Part model, mm, in its own coordinate system. A direction names the side the tool comes from. Round coordinates to 2 decimals unless told otherwise and drop trailing zeros. Write each loop counter-clockwise with the first axis right and the second up, starting at its lowest first coordinate (ties: lowest second). Pieces come first, ordered by that corner, then holes.
from build123d import *

# Parameters (mm, degrees)
SKETCH1_W                        = 15
SKETCH1_H                        = 6
MAIN_BODY_EXT_DEPTH              = 8.3
EMISSION_PATH_EXT_DEPTH          = 9
SKETCH3_R                        = 1.25
EMISSION_AND_GRIN_CUT_DEPTH      = 20.092931
SKETCH4_R                        = 1
DRUM_LENS_CUT_DEPTH              = 13
SKETCH41_R                       = 1
ADDTL_LIGHT_SOURCE_DEPTH         = 5
SKETCH5_W                        = 15
SKETCH5_H                        = 7.3
FILTERCOVER_CUT1_DEPTH           = 1
TOP_LED_SCREW_W                  = 3.06
TOP_LED_SCREW_H                  = 2
BOSS_EXTRUDE1_DEPTH              = 1
FILTERSET_CUT2_DEPTH             = 4
SKETCH10_R                       = 2.5
EMISSION_LENS_CUT_DEPTH          = 8.5
SKETCH15_R                       = 0.795
MAGNETS_CUT_DEPTH                = 0.9
SCREW_HOLES_CUT_DEPTH            = 20.507434
SCREW_HOLES_CUT_DEPTH_BACK       = 2.5
SKETCH18_R                       = 0.375
EXTERNAL_FILLET_1_R              = 1.5
VERTICAL_PATH_CUT_DEPTH          = 14.011149
VERTICAL_PATH_CUT_DEPTH_BACK     = 4
SKETCH28_R                       = 1.5
SET_SCREW_NOTCH_DEPTH            = 3
CUT_EXTRUDE_ORIGINAL_LIGHT_DEPTH = 0.7
CUT_EXTRUDE_ADDTL_LIGHT_DEPTH    = 0.7
SKETCH29_R                       = 0.375
SIDE_LED_SCREW_DEPTH             = 2.5
SKETCH32_W                       = 2
SKETCH32_H                       = 2.36
SIDE_WIRE_SLOT_CUT_DEPTH         = 0.7
SKETCH45_W                       = 2.36
SKETCH45_H                       = 2
TOP_LED_SLOT_DEPTH               = 0.7
CUT_EXTRUDE16_DEPTH              = 9
CUT_EXTRUDE17_REACH              = 13.945
SKETCH37_R                       = 2
SKETCH48_R                       = 0.5
PEG_EXTRUDE_DEPTH                = 2
SKETCH51_R                       = 0.375
TOP_LE_SCREW_DEPTH               = 2.1


with BuildPart() as part:
    # Sketch1 → Main Body Ext (new body)
    with BuildSketch(Plane(origin=(0, 0, 0), x_dir=(1, 0, 0), z_dir=(0, 1, 0))):
        Rectangle(SKETCH1_W, SKETCH1_H)
    extrude(amount=MAIN_BODY_EXT_DEPTH)

    # Sketch8 → Emission Path Ext (add)
    with BuildSketch(Plane(origin=(0, 8.3, 0), x_dir=(1, 0, 0), z_dir=(0, 1, 0))):
        Polygon((-2.75, 3), (-1.5, 1.75), (-1.5, -3), (-7.5, -3), (-7.5, 3), align=None)
    extrude(amount=EMISSION_PATH_EXT_DEPTH)

    # Sketch3 → Emission and Grin Cut (cut, through all)
    with BuildSketch(Plane.XZ):
        with Locations(Location((-4.5, 0, 0), (0, 0, 270))):
            Circle(SKETCH3_R)
    extrude(amount=-EMISSION_AND_GRIN_CUT_DEPTH, mode=Mode.SUBTRACT)

    # Sketch4 → Drum Lens Cut (cut)
    with BuildSketch(Plane(origin=(7.5, 0, 0), x_dir=(0, 0, -1), z_dir=(1, 0, 0))):
        with Locations((0, 3)):
            Circle(SKETCH4_R)
    extrude(amount=-DRUM_LENS_CUT_DEPTH, mode=Mode.SUBTRACT)

    # Sketch41 → Addtl Light Source (cut)
    with BuildSketch(Plane(origin=(0, 8.3, 0), x_dir=(1, 0, 0), z_dir=(0, 1, 0))):
        with Locations(Location((1.5, 0, 0), (0, 0, 270))):
            Circle(SKETCH41_R)
    extrude(amount=-ADDTL_LIGHT_SOURCE_DEPTH, mode=Mode.SUBTRACT)

    # Sketch5 → FilterCover Cut1 (cut)
    with BuildSketch(Plane.XY.offset(3)):
        with Locations((0, 4.65)):
            Rectangle(SKETCH5_W, SKETCH5_H)
    extrude(amount=-FILTERCOVER_CUT1_DEPTH, mode=Mode.SUBTRACT)

    # Top-LED-Screw → Boss-Extrude1 (add)
    with BuildSketch(Plane.XY.offset(2)):
        with Locations((5.97, 7.3)):
            Rectangle(TOP_LED_SCREW_W, TOP_LED_SCREW_H)
    extrude(amount=BOSS_EXTRUDE1_DEPTH)

    # Sketch6 → FilterSet Cut2 (cut)
    with BuildSketch(Plane.XY.offset(2)):
        with BuildLine():
            Line((5.3, 4.5), (5.3, 1.8))
            ThreePointArc((5.3, 1.8), (5.7, 1.4), (5.3, 1))
            Line((5.3, 1), (4.1, 1))
            ThreePointArc((4.1, 1), (3.7, 1.4), (4.1, 1.8))
            Line((4.1, 1.8), (4.1, 4.5))
            ThreePointArc((4.1, 4.5), (4.7, 5.1), (5.3, 4.5))
        make_face()
        with BuildLine():
            Line((-6.9, 7.9), (-6.9, 7.5))
            ThreePointArc((-6.9, 7.5), (-6.782843, 7.217157), (-6.5, 7.1))
            Line((-6.5, 7.1), (-2.5, 7.1))
            ThreePointArc((-2.5, 7.1), (-2.217157, 7.217157), (-2.1, 7.5))
            Line((-2.1, 7.5), (-2.1, 7.9))
            ThreePointArc((-2.1, 7.9), (-2.217157, 8.182843), (-2.5, 8.3))
            Line((-2.5, 8.3), (-6.5, 8.3))
            ThreePointArc((-6.5, 8.3), (-6.782843, 8.182843), (-6.9, 7.9))
        make_face()
        with BuildLine():
            Line((-2.605887, 6.591169), (-6.848528, 2.348528))
            ThreePointArc((-6.848528, 2.348528), (-6.848528, 1.5), (-6, 1.5))
            Line((-6, 1.5), (-1.757359, 5.742641))
            ThreePointArc((-1.757359, 5.742641), (-1.757359, 6.591169), (-2.605887, 6.591169))
        make_face()
        with BuildLine():
            Line((3.112092, 6.591169), (-1.130548, 2.348528))
            ThreePointArc((-1.130548, 2.348528), (-1.130548, 1.5), (-0.28202, 1.5))
            Line((-0.28202, 1.5), (3.96062, 5.742641))
            ThreePointArc((3.96062, 5.742641), (3.96062, 6.591169), (3.112092, 6.591169))
        make_face()
    extrude(amount=-FILTERSET_CUT2_DEPTH, mode=Mode.SUBTRACT)

    # Sketch10 → Emission Lens Cut (cut)
    with BuildSketch(Plane(origin=(0, 17.3, 0), x_dir=(1, 0, 0), z_dir=(0, 1, 0))):
        with Locations(Location((-4.5, 0, 0), (0, 0, 270))):
            Circle(SKETCH10_R)
    extrude(amount=-EMISSION_LENS_CUT_DEPTH, mode=Mode.SUBTRACT)

    # Sketch15 → Magnets Cut (cut)
    with BuildSketch(Plane.XZ):
        with Locations(Location((-6.25, -1.875, 0), (0, 0, 270))):
            Circle(SKETCH15_R)
        with Locations(Location((-6.25, 1.875, 0), (0, 0, 270))):
            Circle(SKETCH15_R)
        with Locations(Location((-1.5, 0, 0), (0, 0, 270))):
            Circle(SKETCH15_R)
    extrude(amount=-MAGNETS_CUT_DEPTH, mode=Mode.SUBTRACT)

    # Sketch18 → Screw Holes Cut (cut, two sides: drawn at the far end of the back side and taken through both)
    with BuildSketch(Plane.XY.offset(2).offset(-SCREW_HOLES_CUT_DEPTH_BACK)):
        with Locations(Location((-6.5, 4, 0), (0, 0, 180))):
            Circle(SKETCH18_R)
        with Locations(Location((6, 5.8, 0), (0, 0, 180))):
            Circle(SKETCH18_R)
        with Locations((0.25, 1)):
            Circle(SKETCH18_R)
    extrude(amount=SCREW_HOLES_CUT_DEPTH + SCREW_HOLES_CUT_DEPTH_BACK, mode=Mode.SUBTRACT)

    # External Fillet 1
    # the kernel refuses this fillet: 1.5 mm, written as the material it takes off along each edge
    with BuildSketch(Plane(origin=(-7.5, -3.75, -3), x_dir=(1, 0, 0), z_dir=(0, 1, 0))) as external_fillet_1_piece_1:
        with BuildLine():
            CenterArc((EXTERNAL_FILLET_1_R, -EXTERNAL_FILLET_1_R), EXTERNAL_FILLET_1_R, 90, 90)
            Line((0, -EXTERNAL_FILLET_1_R), (0, 0))
            Line((0, 0), (EXTERNAL_FILLET_1_R, 0))
        make_face()
    extrude(amount=24.8, mode=Mode.SUBTRACT)
    with BuildSketch(Plane(origin=(-1.5, 8.3, 3), x_dir=(0, 0, -1), z_dir=(0, 1, 0))) as external_fillet_1_piece_2:
        with BuildLine():
            CenterArc((EXTERNAL_FILLET_1_R, EXTERNAL_FILLET_1_R), EXTERNAL_FILLET_1_R, 180, 90)
            Line((0, EXTERNAL_FILLET_1_R), (0, 0))
            Line((0, 0), (EXTERNAL_FILLET_1_R, 0))
        make_face()
    extrude(amount=12.75, mode=Mode.SUBTRACT)

    # Sketch28 → Vertical-Path-Cut (cut, two sides: drawn at the far end of the back side and taken through both)
    with BuildSketch(Plane(origin=(0, 7.1, 0), x_dir=(1, 0, 0), z_dir=(0, 1, 0)).offset(-VERTICAL_PATH_CUT_DEPTH_BACK)):
        with Locations(Location((-4.5, 0, 0), (0, 0, 180))):
            Circle(SKETCH28_R)
    extrude(amount=VERTICAL_PATH_CUT_DEPTH + VERTICAL_PATH_CUT_DEPTH_BACK, mode=Mode.SUBTRACT)

    # Sketch14 → Set-Screw-Notch (cut)
    with BuildSketch(Plane.XZ):
        Polygon((7.5, -3), (7.5, -1.891585), (7.056634, -3), align=None)
    extrude(amount=-SET_SCREW_NOTCH_DEPTH, mode=Mode.SUBTRACT)

    # Sketch12 → Cut-Extrude Original Light (cut)
    with BuildSketch(Plane(origin=(7.5, 0, 0), x_dir=(0, 0, -1), z_dir=(1, 0, 0))):
        with BuildLine():
            Line((1.6, 5.94), (-1.6, 5.94))
            Line((-1.6, 5.94), (-2, 5.94))
            Line((-2, 5.94), (-2, 1.33))
            Line((-2, 1.33), (1.6, 1.33))
            ThreePointArc((1.6, 1.33), (1.882843, 1.447157), (2, 1.73))
            Line((2, 1.73), (2, 5.54))
            ThreePointArc((2, 5.54), (1.882843, 5.822843), (1.6, 5.94))
        make_face()
    extrude(amount=-CUT_EXTRUDE_ORIGINAL_LIGHT_DEPTH, mode=Mode.SUBTRACT)

    # Sketch44 → Cut-Extrude Addtl Light (cut)
    with BuildSketch(Plane(origin=(0, 8.3, 0), x_dir=(1, 0, 0), z_dir=(0, 1, 0))):
        with BuildLine():
            Line((-0.17, -2), (4.44, -2))
            Line((4.44, -2), (4.44, 1.6))
            ThreePointArc((4.44, 1.6), (4.322843, 1.882843), (4.04, 2))
            Line((4.04, 2), (0.23, 2))
            ThreePointArc((0.23, 2), (-0.052843, 1.882843), (-0.17, 1.6))
            Line((-0.17, 1.6), (-0.17, -2))
        make_face()
    extrude(amount=-CUT_EXTRUDE_ADDTL_LIGHT_DEPTH, mode=Mode.SUBTRACT)

    # Sketch29 → Side-LED-Screw (cut)
    with BuildSketch(Plane(origin=(7.5, 0, 0), x_dir=(0, 0, -1), z_dir=(1, 0, 0))):
        with Locations((2, 6.5)):
            Circle(SKETCH29_R)
    extrude(amount=-SIDE_LED_SCREW_DEPTH, mode=Mode.SUBTRACT)

    # Sketch32 → Side-Wire-Slot-Cut (cut)
    with BuildSketch(Plane(origin=(7.5, 0, 0), x_dir=(0, 0, -1), z_dir=(1, 0, 0))):
        with Locations((0, 7.12)):
            Rectangle(SKETCH32_W, SKETCH32_H)
    extrude(amount=-SIDE_WIRE_SLOT_CUT_DEPTH, mode=Mode.SUBTRACT)

    # Sketch45 → Top-LED-slot (cut)
    with BuildSketch(Plane(origin=(0, 8.3, 0), x_dir=(1, 0, 0), z_dir=(0, 1, 0))):
        with Locations((5.62, 0)):
            Rectangle(SKETCH45_W, SKETCH45_H)
    extrude(amount=-TOP_LED_SLOT_DEPTH, mode=Mode.SUBTRACT)

    # Sketch33 → Side-BallLens_Cut (revolve, cut)
    with BuildSketch(Plane.XY, mode=Mode.PRIVATE) as side_balllens_cut_sk:
        with BuildLine():
            Line((6.8, 3), (5.3, 3))
            ThreePointArc((5.3, 3), (5.73934, 4.06066), (6.8, 4.5))
            Line((6.8, 4.5), (6.8, 3))
        make_face()
    revolve(side_balllens_cut_sk.sketch.rotate(Axis((6.8, 3, 0), (-1, 0, 0)), 84.26086), axis=Axis((6.8, 3, 0), (-1, 0, 0)), mode=Mode.SUBTRACT)

    # Sketch47 → Top-BallLens_Cut (revolve, cut)
    with BuildSketch(Plane(origin=(1.5, 0, 0), x_dir=(0, 0, -1), z_dir=(1, 0, 0))):
        with BuildLine():
            Line((-1.5, 7.6), (0, 7.6))
            Line((0, 7.6), (0, 6.137287))
            ThreePointArc((0, 6.137287), (-1.04756, 6.563498), (-1.5, 7.6))
        make_face()
    revolve(axis=Axis((1.5, 7.6, 0), (0, -1, 0)), mode=Mode.SUBTRACT)

    # Sketch36 → Cut-Extrude16 (cut)
    with BuildSketch(Plane(origin=(0, 17.3, 0), x_dir=(1, 0, 0), z_dir=(0, 1, 0))):
        with BuildLine():
            Line((-7.5, -1.5), (-7.5, -3))
            Line((-7.5, -3), (-6, -3))
            ThreePointArc((-6, -3), (-7.06066, -2.56066), (-7.5, -1.5))
        make_face()
    extrude(amount=-CUT_EXTRUDE16_DEPTH, mode=Mode.SUBTRACT)

    # Sketch37 → Cut-Extrude17 (cut, up to next)
    with BuildSketch(Plane(origin=(0, 8.8, 0), x_dir=(1, 0, 0), z_dir=(0, 1, 0)), mode=Mode.PRIVATE) as cut_extrude17_sk1:
        with Locations(Location((-4.5, 0, 0), (0, 0, 180))):
            Circle(SKETCH37_R)
    cut_extrude17_tool1 = extrude(cut_extrude17_sk1.sketch, amount=-CUT_EXTRUDE17_REACH, mode=Mode.PRIVATE) & part.part
    add(cut_extrude17_tool1.solids().sort_by_distance((-4.5, 8.8, 0))[0], mode=Mode.SUBTRACT)

    # Sketch48 → Peg-extrude (cut)
    with BuildSketch(Plane.XZ):
        with Locations(Location((-2, -2, 0), (0, 0, 270))):
            Circle(SKETCH48_R)
    extrude(amount=-PEG_EXTRUDE_DEPTH, mode=Mode.SUBTRACT)

    # Sketch51 → Top-LE-Screw (cut)
    with BuildSketch(Plane(origin=(0, 8.3, 0), x_dir=(1, 0, 0), z_dir=(0, 1, 0))):
        with Locations(Location((5, -2, 0), (0, 0, 270))):
            Circle(SKETCH51_R)
    extrude(amount=-TOP_LE_SCREW_DEPTH, mode=Mode.SUBTRACT)


solid = part.part
Q1. Drop flat-ended pins along their axis: P1, Ø0.6, axis at x = -4, z = 1, coming from the +Y side; P2, Ø2, axis at x = 0.5, z = 1.5, coming from the +Y side; P3, Ø1.6, axis at x = 1.5, z = 0, coming from the +Y side. Give the stop position or say it passes through.
Q2. Saw through at A-A, the plane y = 9.25. Write the cut outline in (x, z).
Q3. Tool access for faces 4 (the flat face through (6, 8.3, 2)), 5 (the flat face through (-2, 2, -2)), 6 (the flat face through (-5, 8, -2)), 7 (the cylindrical face through (-3.073, 4.101, -0.462)): list every direction of +Z, -Z, +X, -X, +Y, -Y with a clear straight run to the whole face (end or side of a thin tool).
Q4. Wall check: line 1 (Z direction, x = 5, y = 7.95) (3 decimals); line 2 (X direction, y = 10, z = 1.5); line 3 (Z direction, x = -4.5, y = 8.5). Give the ranges that are in metal, low to high.
Q5. Two-plate mould, pull along X, no slides. Class faces 1 (the flat face through (7.5, 7, 2)), 2 (the flat face through (-6, 0.9, -2)), 3 (the cylindrical face through (-7.05, 8.53, -2.57)): released by +X, released by -X, zero draft, split by the parting line, or undercut.
Computed:
1. P1: stops at y = 3.1
1. P2: stops at y = 8.3
1. P3: stops at y = 2.4
2. outline: (-7.5, -1.5) arc R1.5 ccw to (-6, -3) - (-2.75, -3) - (-1.5, -1.75) - (-1.5, 1.5) arc R1.5 ccw to (-3, 3) - (-6, 3) arc R1.5 ccw to (-7.5, 1.5) - close; hole circle Ø5 at (-4.5, 0)
3. face 4: +Z, -Z, +X, +Y
3. face 5: -Y
3. face 6: +Z
3. face 7: +Y
4. line 1: z = -3 to -1, 1 to 1.625, 2.375 to 3
4. line 2: x = -7.5 to -6.5, -2.5 to -1.5
4. line 3: z = -3 to -2, 2 to 3
5. face 1: released by +X
5. face 2: undercut
5. face 3: released by -X
